```python
from build123d import *

# Parameters (mm, degrees)
SKETCH1_W           = 70.85
SKETCH1_H           = 16
BOSS_EXTRUDE1_DEPTH = 3
SKETCH2_W           = 8.4
SKETCH2_H           = 16
BOSS_EXTRUDE2_DEPTH = 3
CHAMFER1_SIZE       = 5
CHAMFER1_SIZE2      = 7
SKETCH3_R           = 1.5
CUT_EXTRUDE1_DEPTH  = 3
CHAMFER2_SIZE       = 3
CUT_EXTRUDE2_START  = -3
CUT_EXTRUDE2_DEPTH  = 8
SKETCH5_W           = 3
SKETCH5_H           = 16
BOSS_EXTRUDE3_DEPTH = 8
SKETCH6_R           = 1.5
CUT_EXTRUDE3_DEPTH  = 8
SKETCH7_R           = 1.5
CUT_EXTRUDE4_DEPTH  = 10


with BuildPart() as part:
    # Sketch1 → Boss-Extrude1 (new body)
    with BuildSketch(Plane.XY):
        Rectangle(SKETCH1_W, SKETCH1_H)
    extrude(amount=BOSS_EXTRUDE1_DEPTH)

    # Sketch2 → Boss-Extrude2 (add)
    with BuildSketch(Plane.XY.offset(3)):
        with Locations((-31.225, 0)):
            Rectangle(SKETCH2_W, SKETCH2_H)
    extrude(amount=BOSS_EXTRUDE2_DEPTH)

    # Chamfer1
    chamfer1_edges = [part.edges().sort_by_distance(p)[0] for p in [
        (-35.425, 0, 6),
    ]]
    chamfer1_side = [part.faces().sort_by_distance(p)[0] for p in [
        (-35.425, 0, 3),
    ]]
    chamfer(chamfer1_edges, length=CHAMFER1_SIZE, length2=CHAMFER1_SIZE2, reference=chamfer1_side[0])

    # Sketch3 → Cut-Extrude1 (cut)
    with BuildSketch(Plane(origin=(-12.440878378, 0, 17.41722973), x_dir=(0.8137334712067354, 0, 0.5812381937190957), z_dir=(-0.5812381937190957, 0, 0.8137334712067354))):
        with Locations((-22.642944757, 4)):
            Circle(SKETCH3_R)
        with Locations((-22.642944757, -4)):
            Circle(SKETCH3_R)
    extrude(amount=-CUT_EXTRUDE1_DEPTH, mode=Mode.SUBTRACT)

    # Chamfer2
    chamfer2_edges = [part.edges().sort_by_distance(p)[0] for p in [
        (-27.025, 0, 3),
    ]]
    chamfer(chamfer2_edges, length=CHAMFER2_SIZE - 0.0001)  # a hair under: the kernel refuses the full size

    # Sketch4 → Cut-Extrude2 (cut)
    with BuildSketch(Plane(origin=(-12.440878378, 0, 17.41722973), x_dir=(0.8137334712067354, 0, 0.5812381937190959), z_dir=(-0.5812381937190958, 0, 0.8137334712067353)).offset(CUT_EXTRUDE2_START)):
        Polygon((-19.467518276, 4), (-21.055231516, 6.75), (-24.230657997, 6.75), (-25.818371237, 4), (-24.230657997, 1.25), (-21.055231516, 1.25), align=None)
        Polygon((-19.467518276, -4), (-21.055231516, -1.25), (-24.230657997, -1.25), (-25.818371237, -4), (-24.230657997, -6.75), (-21.055231516, -6.75), align=None)
    extrude(amount=-CUT_EXTRUDE2_DEPTH, mode=Mode.SUBTRACT)

    # Sketch5 → Boss-Extrude3 (add)
    with BuildSketch(Plane.XY.offset(3)):
        with Locations((33.925, 0)):
            Rectangle(SKETCH5_W, SKETCH5_H)
    extrude(amount=BOSS_EXTRUDE3_DEPTH)

    # Sketch6 → Cut-Extrude3 (cut)
    with BuildSketch(Plane(origin=(35.425, 0, 0), x_dir=(0, 0, -1), z_dir=(1, 0, 0))):
        with Locations((-8, 4)):
            Circle(SKETCH6_R)
        with Locations((-8, -4)):
            Circle(SKETCH6_R)
    extrude(amount=-CUT_EXTRUDE3_DEPTH, mode=Mode.SUBTRACT)

    # Sketch7 → Cut-Extrude4 (cut)
    with BuildSketch(Plane(origin=(0, 0, 0), x_dir=(-1, 0, 0), z_dir=(0, 0, -1))):
        with Locations((17.5, 0)):
            Circle(SKETCH7_R)
    extrude(amount=-CUT_EXTRUDE4_DEPTH, mode=Mode.SUBTRACT)


solid = part.part
```
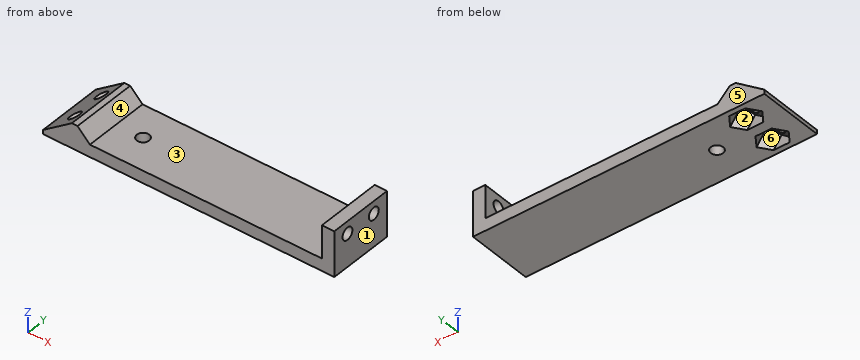
Source: CAD feature listing. Evaluate the final solid. Frame: model axes, mm. Face numbers are marked on the shaded views. A direction names the side the tool comes from. Round coordinates to 2 decimals unless told otherwise and drop trailing zeros. Loops run counter-clockwise (first coordinate to the right, second up) from the corner with the lowest first, then second, coordinate; pieces in that order, holes last.
(1) Section query B-B (z = 8). Output: boundary loops of the cut face in (x, y) (3 decimals), and give its area (3 significant figures).
From the geometry:
outline: (32.425, -8) - (35.425, -8) - (35.425, -5.5) - (32.425, -5.5) - close; (32.425, -2.5) - (35.425, -2.5) - (35.425, 2.5) - (32.425, 2.5) - close; (32.425, 5.5) - (35.425, 5.5) - (35.425, 8) - (32.425, 8) - close
area: 30.0 mm2
(2) Contact query for flat-ended pins moving along their axis: pin 1 Ø2.5 at (y, z) = (-4, 8) entering from -X; pin 2 Ø6 at (y, z) = (2.5, 6.5) entering from -X (3 decimals); pin 3 Ø4 at (y, z) = (-3.5, 6.5) entering from -X; pin 4 Ø3 at (x, y) = (12, -3.5) entering from +Z. Output: stop coordinate, or through.
From the geometry:
pin 1: passes through
pin 2: stops at x = -31.925
pin 3: stops at x = -30.28
pin 4: stops at z = 3
(3) Access query for the marked faces 1, 2 and 3. Directions: +Z, -Z, +X, -X, +Y, -Y. A direction counts if a zero-diameter tool reaches every point of the face in a straight line with its end or side. Return the directions, or none.
From the geometry:
face 1: +Z, -Z, +X, +Y, -Y
face 2: -Z
face 3: +Z, +Y, -Y
(4) Material intervals for probe 1 along Y at (x, z) = (33.3, 8); probe 2 along Y at (x, z) = (-17.5, 0.7); probe 3 along X at (y, z) = (-1, 6.5) (3 decimals), sorted ascending.
From the geometry:
probe 1: y = -8 to -5.5, -2.5 to 2.5, 5.5 to 8
probe 2: y = -8 to -1.5, 1.5 to 8
probe 3: x = 32.425 to 35.425
(5) Section query C-C (x = -17.5). Output: boundary loops of the cut face in (y, z).
From the geometry:
outline: (-8, 0) - (-1.5, 0) - (-1.5, 3) - (-8, 3) - close; (1.5, 0) - (8, 0) - (8, 3) - (1.5, 3) - close
(6) Pull-direction query (Y, two-part tool) for the marked faces 4, 5 and 6; classes: +Y half, -Y half, draft (parallel to the pull), parting line (faces both ways), or undercut.
From the geometry:
face 4: draft
face 5: +Y half
face 6: undercut
(7) Section query D-D (y = -4.75). Give the number of separate pieces and of enclosed holes in the cut face, and give its area (3 significant figures).
From the geometry:
separate pieces: 3
enclosed holes: 0
area: 221 mm2
